```python
from build123d import *

# Parameters (mm, degrees)
F3_D     = 5
F3_DEPTH = 2
F3_TIP   = 1.5021515476
F4_SIZE  = 1.5


with BuildPart() as f1:
    # F0 (on Front) → F1 (revolve)
    with BuildSketch(Plane.XZ):
        Polygon((-120, 0), (0, 0), (0, 5.975), (-100, 5.975), (-100, 7.5), (-108.5, 7.5), (-108.5, 5.975), (-120, 5.975), align=None)
    revolve(axis=Axis((-60, 0, 0), (1, 0, 0)))

    # F3
    with Locations(Plane(origin=(-120, 0, 0), x_dir=(0, -1, 0), z_dir=(-1, 0, 0))):
        with Locations((0, 0)):
            Hole(F3_D / 2, depth=F3_DEPTH)
            with Locations((0, 0, -(F3_DEPTH + F3_TIP / 2))):  # 118° drill point
                Cone(0, F3_D / 2, F3_TIP, mode=Mode.SUBTRACT)

    # F4
    f4_edges = [f1.edges().sort_by_distance(p)[0] for p in [
        (0, 0, -5.975),
    ]]
    chamfer(f4_edges, length=F4_SIZE)


solid = f1.part
```
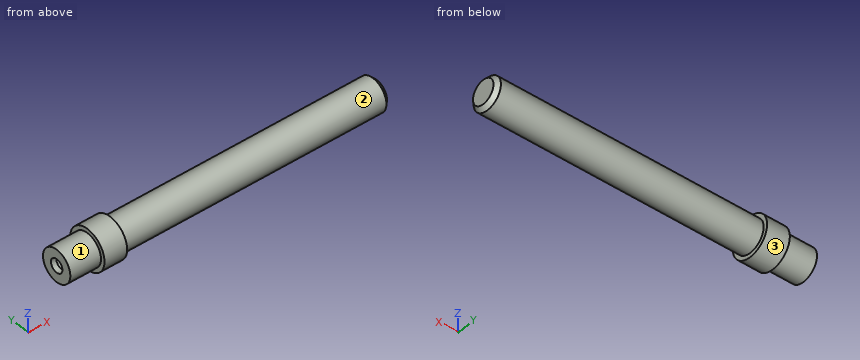
The listing builds one solid part. Answer for the finished solid, in the listing's coordinates (mm). Face numbers are marked on the shaded views. A direction names the side the tool comes from. Give positions to 0.01 mm unless a question says otherwise; leave off trailing zeros. Order: outer loops, then holes, each group sorted by start corner. A loop starts at its lowest first (then second) coordinate and runs counter-clockwise, first axis right, second up. Notation, with made-up numbers: (55, 54) - (107, 54) arc R30 cw to (107, 78) - close; hole circle Ø10 at (-40, 68). An arc over 180 degrees is marked (long way). Use one line per item in the form item = value. Start each with the question number.
(1) Flat-ended cylindrical pins translate along their axes: pin 1 Ø5 at (x, y) = (-50, -2.5) entering from -Z (3 decimals); pin 2 Ø3 at (y, z) = (0, 0) entering from -X. Find the tip coordinate at first contact, or state that the pin passes through.
(2) A cutting plane is placed at A-A, the plane x = -93.5. Write down the section's boundary in (y, z) (3 decimals), then the cut area to 3 significant figures.
(3) For the marked faces 1, 2 and 3, determine the directions among +Z, -Z, +X, -X, +Y, -Y from which every point of the face is accessible in a straight line to the end or side of a thin tool.
(4) Consider line 1 (Z direction, x = -119.45, y = 0) (3 decimals); line 2 (X direction, y = 3, z = -6.5). Determine where each line is inside the solid, lowest interval first. Write a range as from..to.
Ans:
q1.pin_1 = -5.975
q1.pin_2 = -117.4
q2.outline = circle Ø11.95 at (0, 0)
q2.area = 112 mm^2
q3.face_1 = -X
q3.face_2 = +X
q3.face_3 = +X, -X
q4.line_1 = -5.975..-2.5, 2.5..5.975
q4.line_2 = -108.5..-100
